Design review of the part built by this model. Coordinates are the model's own, in mm. A direction names the side the tool comes from. Give positions to 0.01 mm unless a question says otherwise; leave off trailing zeros. Write each loop counter-clockwise with the first axis right and the second up, starting at its lowest first coordinate (ties: lowest second). Pieces come first, ordered by that corner, then holes. Notation, with made-up numbers: (18.5, 13.25) -> (61.5, 13.25) arc R20 cw to (61.5, 48.25) -> close; hole circle Ø8 at (86.5, -38). An arc over 180 degrees is marked (long way). Use CSV: the item, a comma, the result in double quotes.
```python
from build123d import *

# Parameters (mm, degrees)
SKETCH1_R               = 6.35
EXTRUDE1_DEPTH          = 19.05
FILLET1_R               = 12.7
SKETCH2_R               = 52.327921125
CUT_EXTRUDE2_DEPTH      = 12.7
CHAMFER1_SIZE           = 1.27
EXTRUDE2_DEPTH          = 35.56
SKETCH3_R               = 35.56
CUT_EXTRUDE3_DEPTH      = 20.05
CUT_EXTRUDE3_DEPTH_BACK = 36.56
SKETCH5_W               = 101.416551859
SKETCH5_H               = 41.189513353
CUT_EXTRUDE4_DEPTH      = 40.64
SKETCH7_R               = 6.35
CUT_EXTRUDE6_DEPTH      = 36.56


with BuildPart() as part:
    # Sketch1 → Extrude1 (new body)
    with BuildSketch(Plane.XY):
        with BuildLine():
            Line((-60.195770425, 77.931349549), (62.709585641, 77.931349549))
            ThreePointArc((62.709585641, 77.931349549), (90.219330448, 85.014128276), (75.775284214, 60.553520307))
            Line((75.775284214, 60.553520307), (75.775284214, -62.895919466))
            ThreePointArc((75.775284214, -62.895919466), (86.24662402, -89.329307316), (60.199368708, -77.931349549))
            Line((60.199368708, -77.931349549), (-62.691575683, -77.931349549))
            ThreePointArc((-62.691575683, -77.931349549), (-90.218375384, -84.744460999), (-75.775284214, -60.340766466))
            Line((-75.775284214, -60.340766466), (-75.775284214, 62.510464201))
            ThreePointArc((-75.775284214, 62.510464201), (-86.384477207, 88.809119355), (-60.195770425, 77.931349549))
        make_face()
        with Locations((77.931349549, 75.775284214)):
            Circle(SKETCH1_R, mode=Mode.SUBTRACT)
        with Locations((75.775284214, -77.931349549)):
            Circle(SKETCH1_R, mode=Mode.SUBTRACT)
        with Locations((-77.931349549, -75.775284214)):
            Circle(SKETCH1_R, mode=Mode.SUBTRACT)
        with Locations((-75.775284214, 77.931349549)):
            Circle(SKETCH1_R, mode=Mode.SUBTRACT)
    extrude(amount=EXTRUDE1_DEPTH)

    # Fillet1
    fillet1_edges = [part.edges().sort_by_distance(p)[0] for p in [
        (-75.775284214, -60.340766466, 9.525),
        (-75.775284214, 62.510464201, 9.525),
        (-60.195770425, 77.931349549, 9.525),
        (62.709585641, 77.931349549, 9.525),
        (75.775284214, 60.553520307, 9.525),
        (75.775284214, -62.895919466, 9.525),
        (60.199368708, -77.931349549, 9.525),
        (-62.691575683, -77.931349549, 9.525),
    ]]
    fillet(fillet1_edges, radius=FILLET1_R)

    # Sketch2 → Cut-Extrude2 (cut)
    with BuildSketch(Plane.XY.offset(19.05)):
        Circle(SKETCH2_R)
    extrude(amount=-CUT_EXTRUDE2_DEPTH, mode=Mode.SUBTRACT)

    # Chamfer1
    chamfer1_edges = [part.edges().sort_by_distance(p)[0] for p in [
        (-52.327921125, 0, 19.05),
    ]]
    chamfer(chamfer1_edges, length=CHAMFER1_SIZE)

    # Sketch4 → Extrude2 (add)
    with BuildSketch(Plane(origin=(0, 0, 0), x_dir=(-1, 0, 0), z_dir=(0, 0, -1))):
        with BuildLine():
            Line((86.089983669, -49.856504988), (99.397574405, -57.563208318))
            ThreePointArc((99.397574405, -57.563208318), (104.035719005, -62.2105938), (105.732985822, -68.553295314))
            Line((105.732985822, -68.553295314), (105.732985822, -88.945536156))
            ThreePointArc((105.732985822, -88.945536156), (102.013241943, -97.925792277), (93.032985822, -101.645536156))
            Line((93.032985822, -101.645536156), (-93.521645158, -101.645536156))
            ThreePointArc((-93.521645158, -101.645536156), (-102.501901279, -97.925792277), (-106.221645158, -88.945536156))
            Line((-106.221645158, -88.945536156), (-106.221645158, -65.233714494))
            ThreePointArc((-106.221645158, -65.233714494), (-105.262508623, -61.659777941), (-102.642852051, -59.046281274))
            Line((-102.642852051, -59.046281274), (-86.23402563, -49.606947108))
            ThreePointArc((-86.23402563, -49.606947108), (-80.539133122, -42.676006174), (-80.844982944, -33.710728777))
            ThreePointArc((-80.844982944, -33.710728777), (0.126849431, 87.591714284), (80.747004975, -33.944744652))
            ThreePointArc((80.747004975, -33.944744652), (80.415189643, -42.909098588), (86.089983669, -49.856504988))
        make_face()
    extrude(amount=EXTRUDE2_DEPTH)

    # Sketch3 → Cut-Extrude3 (cut, two sides)
    with BuildSketch(Plane.XY) as cut_extrude3_sk:
        Circle(SKETCH3_R)
    extrude(amount=CUT_EXTRUDE3_DEPTH, mode=Mode.SUBTRACT)
    extrude(cut_extrude3_sk.sketch, amount=-CUT_EXTRUDE3_DEPTH_BACK, mode=Mode.SUBTRACT)

    # Sketch5 → Cut-Extrude4 (cut)
    with BuildSketch(Plane.XY):
        with Locations((-2.36196921, 98.526106226)):
            Rectangle(SKETCH5_W, SKETCH5_H)
    extrude(amount=-CUT_EXTRUDE4_DEPTH, mode=Mode.SUBTRACT)

    # Sketch7 → Cut-Extrude6 (cut, through all)
    with BuildSketch(Plane.XY):
        with Locations((75.775284214, -77.931349549)):
            Circle(SKETCH7_R)
        with Locations((-77.931349549, -75.775284214)):
            Circle(SKETCH7_R)
    extrude(amount=-CUT_EXTRUDE6_DEPTH, mode=Mode.SUBTRACT)


solid = part.part
```
(1) Take a section at B-B (x = 0). Write out the cut boundary in (y, z).
Established:
outline,"(-101.65, -35.56) -> (-35.56, -35.56) -> (-35.56, 6.35) -> (-52.33, 6.35) -> (-52.33, 17.78) -> (-53.6, 19.05) -> (-77.93, 19.05) -> (-77.93, 0) -> (-101.65, 0) -> close; (35.56, -35.56) -> (77.93, -35.56) -> (77.93, 19.05) -> (53.6, 19.05) -> (52.33, 17.78) -> (52.33, 6.35) -> (35.56, 6.35) -> close"
(2) Clearance check with flat-ended pins moving along their axes: pin 1 (16.5 mm diameter, centred on x = 9, z = 0, fed in from +Y); pin 2 (6 mm diameter, centred on y = 17, z = -2.5, fed in from +X); pin 3 (10 mm diameter, centred on x = -84.5, z = -15.5, fed in from +Y). State where each tip first meets the part, or that it passes through.
Established:
pin 1,"stops at y = 77.93"
pin 2,"stops at x = 86.47"
pin 3,"stops at y = 36.77"
(3) Take a section at C-C (z = -28). Write out the cut boundary in (x, y).
Established:
outline,"(-105.73, -88.95) arc R12.7 ccw to (-93.03, -101.65) -> (93.52, -101.65) arc R12.7 ccw to (106.22, -88.95) -> (106.22, -65.23) arc R7.14 ccw to (102.64, -59.05) -> (86.23, -49.61) arc R12.7 cw to (80.84, -33.71) arc R87.59 ccw to (39.99, 77.93) -> (-39.99, 77.93) arc R87.59 ccw to (-80.75, -33.94) arc R12.7 cw to (-86.09, -49.86) -> (-99.4, -57.56) arc R12.7 ccw to (-105.73, -68.55) -> close; hole circle Ø12.7 at (-77.93, -75.78); hole circle Ø71.12 at (0, 0); hole circle Ø12.7 at (75.78, -77.93)"
(4) Tool access review of faces 1 (the face through (-1, -77.931, 9)), 2 (the face through (34, -11, 6.35)), 3 (the face through (-77.68, 59.64, 9.66)), 4 (the face through (-75.775, 1, 9)): name each direction out of +Z, -Z, +X, -X, +Y, -Y from which nothing blocks a thin tool from reaching the whole face with its end or side.
Established:
face 1,"+Z, -Y"
face 2,"+Z"
face 3,"+Z, -Z, -X"
face 4,"+Z, -X"
(5) For line 1 along Y through (x, z) = (0, 13); line 2 along X through (y, z) = (-79.5, 10.5); line 3 along Y through (x, z) = (74, 12), list the stretches that pass through material, from the lowest coordinate up. Write a range as [from, to].
Established:
line 1,"y = [-77.93, -52.33], [52.33, 77.93]"
line 2,"x = [-92.75, -83.07], [-72.79, -60.31], [56.48, 69.62], [81.93, 90.89]"
line 3,"y = [-93.56, -84.03], [-71.83, 70.79], [80.76, 90.64]"
(6) Take a section at A-A (y = 0). Write out the cut boundary in (x, z).
Established:
outline,"(-87.59, -35.56) -> (-35.56, -35.56) -> (-35.56, 6.35) -> (-52.33, 6.35) -> (-52.33, 17.78) -> (-53.6, 19.05) -> (-75.78, 19.05) -> (-75.78, 0) -> (-87.59, 0) -> close; (35.56, -35.56) -> (87.59, -35.56) -> (87.59, 0) -> (75.78, 0) -> (75.78, 19.05) -> (53.6, 19.05) -> (52.33, 17.78) -> (52.33, 6.35) -> (35.56, 6.35) -> close"
